Build history of the part. All positions in model axes, mm. Face numbers are marked on the shaded views. A direction names the side the tool comes from. Give positions to 0.01 mm unless a question says otherwise; leave off trailing zeros. Loops run counter-clockwise (first coordinate to the right, second up) from the corner with the lowest first, then second, coordinate; pieces in that order, holes last. Notation, with made-up numbers: (35.5, -15.75) -> (73.5, -15.75) arc R22 ccw to (73.5, 15.25) -> close; hole circle Ø2 at (15, 35.5). An arc over 180 degrees is marked (long way). Answer in a Markdown table with one row per item. Add a question column.
from build123d import *

# Parameters (mm, degrees)
F1_DEPTH = 10
F3_DEPTH = 3


with BuildPart() as f1:
    # F0 (on Top) → F1 (new body)
    with BuildSketch(Plane.XY):
        with BuildLine():
            Line((81.289, 10), (0, 10))
            ThreePointArc((0, 10), (-7.071068, 7.071068), (-10, 0))
            Line((-10, 0), (-10, -26.108))
            Line((-10, -26.108), (-10, -52.216))
            ThreePointArc((-10, -52.216), (-7.071068, -59.287068), (0, -62.216))
            Line((0, -62.216), (81.289, -62.216))
            ThreePointArc((81.289, -62.216), (88.360068, -59.287068), (91.289, -52.216))
            Line((91.289, -52.216), (91.289, -26.108))
            Line((91.289, -26.108), (91.289, 0))
            ThreePointArc((91.289, 0), (88.360068, 7.071068), (81.289, 10))
        make_face()
        with BuildLine():
            ThreePointArc((3.570714, -55.716), (-5, -52.216), (3.570714, -48.716))
            Line((3.570714, -48.716), (4.728286, -48.716))
            ThreePointArc((4.728286, -48.716), (8.299, -47.216), (11.869714, -48.716))
            Line((11.869714, -48.716), (19.625286, -48.716))
            ThreePointArc((19.625286, -48.716), (23.196, -47.216), (26.766714, -48.716))
            Line((26.766714, -48.716), (27.924286, -48.716))
            ThreePointArc((27.924286, -48.716), (31.495, -47.216), (35.065714, -48.716))
            Line((35.065714, -48.716), (36.223286, -48.716))
            ThreePointArc((36.223286, -48.716), (39.794, -47.216), (43.364714, -48.716))
            Line((43.364714, -48.716), (46.223286, -48.716))
            ThreePointArc((46.223286, -48.716), (49.794, -47.216), (53.364714, -48.716))
            Line((53.364714, -48.716), (54.522286, -48.716))
            ThreePointArc((54.522286, -48.716), (58.093, -47.216), (61.663714, -48.716))
            Line((61.663714, -48.716), (69.419286, -48.716))
            ThreePointArc((69.419286, -48.716), (72.99, -47.216), (76.560714, -48.716))
            Line((76.560714, -48.716), (77.718286, -48.716))
            ThreePointArc((77.718286, -48.716), (83.179295, -47.587092), (86.289, -52.216))
            ThreePointArc((86.289, -52.216), (83.179295, -56.844908), (77.718286, -55.716))
            Line((77.718286, -55.716), (76.560714, -55.716))
            ThreePointArc((76.560714, -55.716), (72.99, -57.216), (69.419286, -55.716))
            Line((69.419286, -55.716), (61.663714, -55.716))
            ThreePointArc((61.663714, -55.716), (58.093, -57.216), (54.522286, -55.716))
            Line((54.522286, -55.716), (53.364714, -55.716))
            ThreePointArc((53.364714, -55.716), (49.794, -57.216), (46.223286, -55.716))
            Line((46.223286, -55.716), (43.364714, -55.716))
            ThreePointArc((43.364714, -55.716), (39.794, -57.216), (36.223286, -55.716))
            Line((36.223286, -55.716), (35.065714, -55.716))
            ThreePointArc((35.065714, -55.716), (31.495, -57.216), (27.924286, -55.716))
            Line((27.924286, -55.716), (26.766714, -55.716))
            ThreePointArc((26.766714, -55.716), (23.196, -57.216), (19.625286, -55.716))
            Line((19.625286, -55.716), (11.869714, -55.716))
            ThreePointArc((11.869714, -55.716), (8.299, -57.216), (4.728286, -55.716))
            Line((4.728286, -55.716), (3.570714, -55.716))
        make_face(mode=Mode.SUBTRACT)
        Polygon((0, -42.216), (0, -26.108), (0, -10), (81.289, -10), (81.289, -26.108), (81.289, -42.216), align=None, mode=Mode.SUBTRACT)
        with BuildLine():
            ThreePointArc((3.570714, -3.5), (-5, 0), (3.570714, 3.5))
            Line((3.570714, 3.5), (4.728286, 3.5))
            ThreePointArc((4.728286, 3.5), (8.299, 5), (11.869714, 3.5))
            Line((11.869714, 3.5), (19.625286, 3.5))
            ThreePointArc((19.625286, 3.5), (23.196, 5), (26.766714, 3.5))
            Line((26.766714, 3.5), (27.924286, 3.5))
            ThreePointArc((27.924286, 3.5), (31.495, 5), (35.065714, 3.5))
            Line((35.065714, 3.5), (46.223286, 3.5))
            ThreePointArc((46.223286, 3.5), (49.794, 5), (53.364714, 3.5))
            Line((53.364714, 3.5), (54.522286, 3.5))
            ThreePointArc((54.522286, 3.5), (58.093, 5), (61.663714, 3.5))
            Line((61.663714, 3.5), (69.419286, 3.5))
            ThreePointArc((69.419286, 3.5), (72.99, 5), (76.560714, 3.5))
            Line((76.560714, 3.5), (77.718286, 3.5))
            ThreePointArc((77.718286, 3.5), (83.179295, 4.628908), (86.289, 0))
            ThreePointArc((86.289, 0), (83.179295, -4.628908), (77.718286, -3.5))
            Line((77.718286, -3.5), (76.560714, -3.5))
            ThreePointArc((76.560714, -3.5), (72.99, -5), (69.419286, -3.5))
            Line((69.419286, -3.5), (61.663714, -3.5))
            ThreePointArc((61.663714, -3.5), (58.093, -5), (54.522286, -3.5))
            Line((54.522286, -3.5), (53.364714, -3.5))
            ThreePointArc((53.364714, -3.5), (49.794, -5), (46.223286, -3.5))
            Line((46.223286, -3.5), (35.065714, -3.5))
            ThreePointArc((35.065714, -3.5), (31.495, -5), (27.924286, -3.5))
            Line((27.924286, -3.5), (26.766714, -3.5))
            ThreePointArc((26.766714, -3.5), (23.196, -5), (19.625286, -3.5))
            Line((19.625286, -3.5), (11.869714, -3.5))
            ThreePointArc((11.869714, -3.5), (8.299, -5), (4.728286, -3.5))
            Line((4.728286, -3.5), (3.570714, -3.5))
        make_face(mode=Mode.SUBTRACT)
    extrude(amount=F1_DEPTH)

    # F2 (on face) → F3 (join)
    with BuildSketch(Plane(origin=(0, 0, 0), x_dir=(1, 0, 0), z_dir=(0, 0, -1))):
        with BuildLine():
            ThreePointArc((0, 62.216), (-7.071068, 59.287068), (-10, 52.216))
            Line((-10, 52.216), (-10, 0))
            ThreePointArc((-10, 0), (-7.071068, -7.071068), (0, -10))
            Line((0, -10), (81.289, -10))
            ThreePointArc((81.289, -10), (88.360068, -7.071068), (91.289, 0))
            Line((91.289, 0), (91.289, 52.216))
            ThreePointArc((91.289, 52.216), (88.360068, 59.287068), (81.289, 62.216))
            Line((81.289, 62.216), (0, 62.216))
        make_face()
    extrude(amount=F3_DEPTH)


solid = f1.part
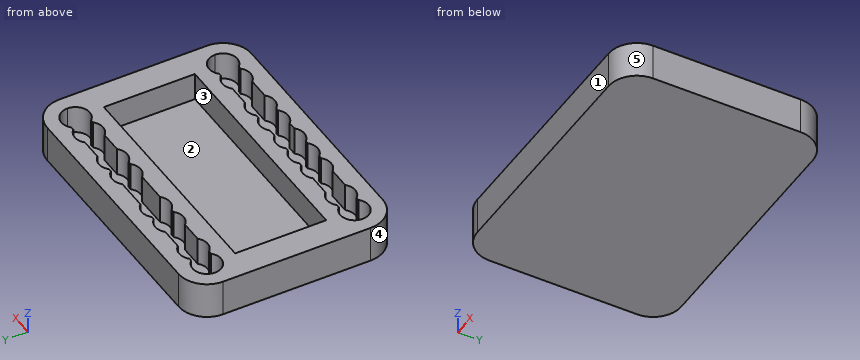
(1) Flat gauge pin, fed straight in: pin 1 Ø5 at (x, y) = (19.5, -27) entering from +Z. Where does the tip first touch, or does it go through?
(2) Saw through at D-D, the plane x = 33. List the corners of the cut face in (y, z).
(3) Saw through at B-B, the plane x = 64.5. List the corners of the cut face in (y, z), then the cut area to 3 significant figures.
(4) Saw through at C-C, the plane z = 4.5. State how many separate pieces and enclosed holes the cut face has, then the cut area to 3 significant figures.
(5) 3-axis set-ups, long thin cutter, end or side, ignore diameter. For the marked faces 1 and 2: which of +Z, -Z, +X, -X, +Y, -Y reach the whole face in a straight line?
(6) Two-plate mould, pull along X, no slides. Class the marked faces 3, 4 and 5: released by +X, released by -X, zero draft, split by the parting line, or undercut.
(7) Saw through at A-A, the plane y = -30. List the corners of the cut face in (x, z), then the cut area to 3 significant figures.
(8) Wall check: line 1 along Y through (x, z) = (81, 7); line 2 along Y through (x, z) = (16, 4); line 3 along X through (y, z) = (-40.5, 7.5). Give the ranges that are in metal, low to high. Write a range as from..to.
Worked answers:
| question | item | result |
|---|---|---|
| 1 | pin 1 | z = 0 |
| 2 | outline | (-62.22, -3) -> (10, -3) -> (10, 10) -> (4.77, 10) -> (4.77, 0) -> (-4.77, 0) -> (-4.77, 10) -> (-10, 10) -> (-10, 0) -> (-42.22, 0) -> (-42.22, 10) -> (-47.45, 10) -> (-47.45, 0) -> (-56.98, 0) -> (-56.98, 10) -> (-62.22, 10) -> close |
| 3 | outline | (-62.22, -3) -> (10, -3) -> (10, 10) -> (3.5, 10) -> (3.5, 0) -> (-3.5, 0) -> (-3.5, 10) -> (-10, 10) -> (-10, 0) -> (-42.22, 0) -> (-42.22, 10) -> (-48.72, 10) -> (-48.72, 0) -> (-55.72, 0) -> (-55.72, 10) -> (-62.22, 10) -> close |
| 3 | area | 477 mm^2 |
| 4 | separate pieces | 1 |
| 4 | enclosed holes | 3 |
| 4 | area | 3,090 mm^2 |
| 5 | face 1 | +Z, -Z, +X, -X, -Y |
| 5 | face 2 | +Z |
| 6 | face 3 | undercut |
| 6 | face 4 | released by -X |
| 6 | face 5 | released by +X |
| 7 | outline | (-10, -3) -> (91.29, -3) -> (91.29, 10) -> (81.29, 10) -> (81.29, 0) -> (0, 0) -> (0, 10) -> (-10, 10) -> close |
| 7 | area | 504 mm^2 |
| 8 | line 1 | -62.22..-57.21, -47.22..-42.22, -10..-4.99, 4.99..10 |
| 8 | line 2 | -62.22..-55.72, -48.72..-42.22, -10..-3.5, 3.5..10 |
| 8 | line 3 | -10..0, 81.29..91.29 |
